from build123d import *

# Parameters (mm, degrees)
F0_W     = 58.42
F0_H     = 38.1
F1_DEPTH = 12.7
F2_R     = 6.985
F3_DEPTH = 19.05


with BuildPart() as f1:
    # F0 (on Top) → F1 (new body)
    with BuildSketch(Plane.XY):
        Rectangle(F0_W, F0_H)
    extrude(amount=-F1_DEPTH)

    # F2 (on face) → F3 (join)
    with BuildSketch(Plane.YZ.offset(29.21)):
        with BuildLine():
            Line((-19.05, 0), (19.05, 0))
            Line((19.05, 0), (19.05, 50.8))
            ThreePointArc((19.05, 50.8), (0, 69.85), (-19.05, 50.8))
            Line((-19.05, 50.8), (-19.05, 0))
        make_face()
        with Locations((0, 50.8)):
            Circle(F2_R, mode=Mode.SUBTRACT)
    extrude(amount=-F3_DEPTH)

    # F4: F1 across plane


with BuildPart() as f1_1:
    add(f1.part)
    add(f1.part.mirror(Plane.YZ))


solid = f1_1.part
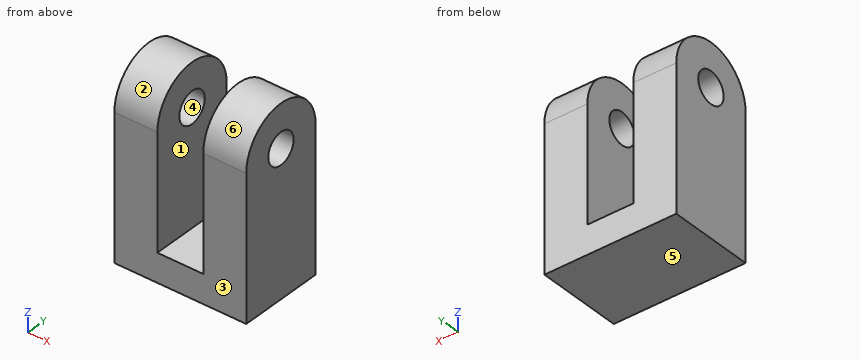
Model file for the job. Use its own axes, mm. Face numbers are marked on the shaded views. A direction names the side the tool comes from. Round coordinates to 2 decimals unless told otherwise and drop trailing zeros. Order: outer loops, then holes, each group sorted by start corner. A loop starts at its lowest first (then second) coordinate and runs counter-clockwise, first axis right, second up.
(1) Pin check, flat tips, straight feed: pin 1 (10 mm diameter, centred on x = -5, y = -12.5, fed in from +Z); pin 2 (10 mm diameter, centred on x = -15, y = 6, fed in from +Z); pin 3 (12.5 mm diameter, centred on y = 0, z = 50.8, fed in from -X); pin 4 (18 mm diameter, centred on y = 0, z = 50.8, fed in from -X). Stop position of each tip, or through.
(2) Band-saw the part on D-D (z = 55). List the corners of the cut face in (x, y), then the cut area to 3 significant figures.
(3) Pull direction Z, two halves, no side cores. Call the marked faces 3, 4, 5 and 6: released by +Z, released by -Z, zero draft, split by the parting line, or undercut.
(4) Drill centre lines: line 1 (X direction, y = -0.5, z = 4.5); line 2 (Z direction, x = -16.25, y = 0) (3 decimals); line 3 (Y direction, x = 19, z = 51). Where is each one in solid material? Low to high.
(5) Band-saw the part on B-B (z = 28). List the corners of the cut face in (x, y).
(6) 3-axis set-ups, long thin cutter, end or side, ignore diameter. For the marked faces 1 and 2: which of +Z, -Z, +X, -X, +Y, -Y reach the whole face in a straight line?
(7) Band-saw the part on A-A (y = 0). List the corners of the cut face in (x, z) (3 decimals).
(8) Band-saw the part on C-C (x = -18.5). List the corners of the cut face in (y, z) (3 decimals), then the cut area to 3 significant figures.
Verdict:
1. pin 1: stops at z = 0
1. pin 2: stops at z = 69.82
1. pin 3: passes through
1. pin 4: stops at x = -29.21
2. outline: (-29.21, -18.58) - (-10.16, -18.58) - (-10.16, -5.58) - (-29.21, -5.58) - close; (-29.21, 5.58) - (-10.16, 5.58) - (-10.16, 18.58) - (-29.21, 18.58) - close; (10.16, -18.58) - (29.21, -18.58) - (29.21, -5.58) - (10.16, -5.58) - close; (10.16, 5.58) - (29.21, 5.58) - (29.21, 18.58) - (10.16, 18.58) - close
2. area: 991 mm2
3. face 3: zero draft
3. face 4: undercut
3. face 5: released by -Z
3. face 6: released by +Z
4. line 1: x = -29.21 to -10.16, 10.16 to 29.21
4. line 2: z = -12.7 to 43.815, 57.785 to 69.85
4. line 3: y = -19.05 to -6.98, 6.98 to 19.05
5. outline: (-29.21, -19.05) - (-10.16, -19.05) - (-10.16, 19.05) - (-29.21, 19.05) - close; (10.16, -19.05) - (29.21, -19.05) - (29.21, 19.05) - (10.16, 19.05) - close
6. face 1: +Z, +Y, -Y
6. face 2: +Z, +X, -X
7. outline: (-29.21, -12.7) - (29.21, -12.7) - (29.21, 43.815) - (10.16, 43.815) - (10.16, 0) - (-10.16, 0) - (-10.16, 43.815) - (-29.21, 43.815) - close; (-29.21, 57.785) - (-10.16, 57.785) - (-10.16, 69.85) - (-29.21, 69.85) - close; (10.16, 57.785) - (29.21, 57.785) - (29.21, 69.85) - (10.16, 69.85) - close
8. outline: (-19.05, -12.7) - (19.05, -12.7) - (19.05, 50.8) arc R19.05 ccw to (-19.05, 50.8) - close; hole circle Ø13.97 at (0, 50.8)
8. area: 2,840 mm2
